from build123d import *

# Parameters (mm, degrees)
F1_DEPTH = 12
F2_R     = 1.75
F3_DEPTH = 19.151
F4_SIZE  = 1.5
F5_W     = 8.5
F5_H     = 2.4
F6_DEPTH = 1.2
F7_W     = 8.5
F7_H     = 2.4
F8_DEPTH = 1.2
F9_SIZE  = 1.19999


# Not quite as in the source:
# - a fillet or chamfer is up to 0.001 mm smaller than in the source, because OpenCascade refuses the exact size


with BuildPart() as f1:
    # F0 (on Front) → F1 (new body)
    with BuildSketch(Plane.XZ):
        with BuildLine():
            Line((-35.8277369916, 41.9945976296), (-39.0277369916, 41.9945976296))
            Line((-39.0277369916, 41.9945976296), (-39.0277369916, 27.5945976296))
            Line((-39.0277369916, 27.5945976296), (-30.5277369916, 27.5945976296))
            ThreePointArc((-30.5277369916, 27.5945976296), (-22.2777369916, 19.3445976296), (-30.5277369916, 11.0945976296))
            Line((-30.5277369916, 11.0945976296), (-39.0277369916, 11.0945976296))
            Line((-39.0277369916, 11.0945976296), (-39.0277369916, -3.3054023704))
            Line((-39.0277369916, -3.3054023704), (-35.8277369916, -3.3054023704))
            Line((-35.8277369916, -3.3054023704), (-35.8277369916, 8.6945976296))
            Line((-35.8277369916, 8.6945976296), (-30.5277369916, 8.6945976296))
            ThreePointArc((-30.5277369916, 8.6945976296), (-19.8777369916, 19.3445976296), (-30.5277369916, 29.9945976296))
            Line((-30.5277369916, 29.9945976296), (-35.8277369916, 29.9945976296))
            Line((-35.8277369916, 29.9945976296), (-35.8277369916, 41.9945976296))
        make_face()
    extrude(amount=F1_DEPTH)

    # F2 (on face) → F3 (cut, through all)
    with BuildSketch(Plane(origin=(-39.0277369916, 0, 0), x_dir=(0, -1, 0), z_dir=(-1, 0, 0))):
        with Locations((6, 35.9945976296)):
            Circle(F2_R)
        with Locations((6, 2.6945976296)):
            Circle(F2_R)
    extrude(amount=-F3_DEPTH, mode=Mode.SUBTRACT)

    # F4
    f4_edges = [f1.edges().sort_by_distance(p)[0] for p in [
        (-35.827737, -4.25, 35.994598),
        (-35.827737, -4.25, 2.694598),
    ]]
    chamfer(f4_edges, length=F4_SIZE)

    # F5 (on face) → F6 (join)
    with BuildSketch(Plane.XY.offset(11.0945976296)):
        with Locations((-34.7777369916, -6)):
            Rectangle(F5_W, F5_H)
    extrude(amount=F6_DEPTH)

    # F7 (on face) → F8 (join)
    with BuildSketch(Plane(origin=(0, 0, 27.5945976296), x_dir=(1, 0, 0), z_dir=(0, 0, -1))):
        with Locations((-34.7777369916, 6)):
            Rectangle(F7_W, F7_H)
    extrude(amount=F8_DEPTH)

    # F9 (size 1.2 in the source; OpenCascade refuses exactly that, so slightly less here)
    f9_edges = [f1.edges().sort_by_distance(p)[0] for p in [
        (-34.777737, -7.2, 12.294598),
        (-34.777737, -4.8, 12.294598),
        (-34.777737, -7.2, 26.394598),
        (-34.777737, -4.8, 26.394598),
    ]]
    chamfer(f9_edges, length=F9_SIZE)


solid = f1.part
Geometry check sheet. Reference: the model listing, model coordinates, mm. A direction names the side the tool comes from. Give positions to 0.01 mm unless a question says otherwise; leave off trailing zeros. Loops run counter-clockwise (first coordinate to the right, second up) from the corner with the lowest first, then second, coordinate; pieces in that order, holes last. Notation, with made-up numbers: (55, 25) -> (62, 25) arc R24 cw to (62, 55) -> close; hole circle Ø5 at (-15, 33). An arc over 180 degrees is marked (long way). Answer in a Markdown table with one row per item. Add a question column.
1) Cross-section at B-B on y = -1.5. Record the boundary of the cut face in (x, z), and give its area (3 significant figures).
2) Set-up check for faces 1 (the face through (-33, -6, 29.995)), 2 (the face through (-34.837, -6.608, 11.686)), 3 (the face through (-35.828, -3, 5)), 4 (the face through (-34.837, -5.408, 11.703)): record each of +Z, -Z, +X, -X, +Y, -Y from which the full face is reachable in a straight line by a thin tool's end or side.
3) Cross-section at C-C on x = -28.25. Record the boundary of the cut face in (y, z).
4) Material ranges on probe 1 along Z at (x, y) = (-35.25, -0.75); probe 2 along X at (y, z) = (-4, 39.5); probe 3 along Z at (x, y) = (-27.25, -3.5), recorded low to high. Write a range as from..to.
5) Gauge pin test, flat ends, axial feed: P1, Ø5.5, axis at y = -6, z = 2.69, coming from the +X side; P2, Ø1.5, axis at x = -31, y = -8.5, coming from the +Z side; P3, Ø6, axis at x = -35.5, z = 24, coming from the +Y side. Record the tip position at first contact, or that the pin passes through.
6) Draft check along Y on faces 5 (the face through (-34.837, -5.408, 26.986)), 6 (the face through (-39.028, -5, 34)), 7 (the face through (-38.19, -5.77, 37.73)). Enter one of: pulls with the +Y half, pulls with the -Y half, needs draft (parallel to the pull), parting line crosses it, or undercut.
7) Cross-section at D-D on z = 19. Record the boundary of the cut face in (x, y), and give its area (3 significant figures).
Outcome:
| question | item | result |
|---|---|---|
| 1 | outline | (-39.03, -3.31) -> (-35.83, -3.31) -> (-35.83, 8.69) -> (-30.53, 8.69) arc R10.65 ccw to (-30.53, 29.99) -> (-35.83, 29.99) -> (-35.83, 41.99) -> (-39.03, 41.99) -> (-39.03, 27.59) -> (-30.53, 27.59) arc R8.25 cw to (-30.53, 11.09) -> (-39.03, 11.09) -> close |
| 1 | area | 189 mm^2 |
| 2 | face 1 | +Z, +X, +Y, -Y |
| 2 | face 2 | -X, -Y |
| 2 | face 3 | -Z, +X, +Y, -Y |
| 2 | face 4 | -X, +Y |
| 3 | outline | (-12, 8.94) -> (0, 8.94) -> (0, 11.42) -> (-12, 11.42) -> close; (-12, 27.27) -> (0, 27.27) -> (0, 29.75) -> (-12, 29.75) -> close |
| 4 | probe 1 | z = 8.69..11.09, 27.59..29.99 |
| 4 | probe 2 | x = -39.03..-35.83 |
| 4 | probe 3 | z = 9.21..11.77, 26.92..29.48 |
| 5 | P1 | stops at x = -36.32 |
| 5 | P2 | stops at z = 29.99 |
| 5 | P3 | stops at y = -5.39 |
| 6 | face 5 | pulls with the +Y half |
| 6 | face 6 | needs draft |
| 6 | face 7 | undercut |
| 7 | outline | (-22.28, -12) -> (-19.88, -12) -> (-19.88, 0) -> (-22.28, 0) -> close |
| 7 | area | 28.8 mm^2 |
